```python
from build123d import *

# Parameters (mm, degrees)
F1_DEPTH = 25.4
F2_R     = 2.486175
F3_DEPTH = 25.4


with BuildPart() as f1:
    # F0 (on Top) → F1 (new body)
    with BuildSketch(Plane.XY):
        Polygon((-25.4, 0), (0, 0), (-25.4, 33.05722), align=None)
    extrude(amount=F1_DEPTH)

    # F2 (on face) → F3 (join)
    with BuildSketch(Plane.XY.offset(25.4)):
        with Locations((-16.399799, 11.118355)):
            Circle(F2_R)
    extrude(amount=F3_DEPTH)


solid = f1.part
```
Work out the finished part from the listing and answer in its coordinate system (mm). Give positions to 0.01 mm unless a question says otherwise; leave off trailing zeros. Loops run counter-clockwise (first coordinate to the right, second up) from the corner with the lowest first, then second, coordinate; pieces in that order, holes last. Notation, with made-up numbers: (-6.5, 63) - (14.5, 63) arc R13 cw to (14.5, 75) - close; hole circle Ø6 at (88, -22.5). An arc over 180 degrees is marked (long way). Use CSV: the item, a comma, the result in double quotes. Start each with the question number.
(1) Find section A-A, the plane y = 10. Determine the outline of the cut face in (x, z), plus the area to 3 significant figures.
(2) Find section D-D, the plane y = 21. Determine the outline of the cut face in (x, z), plus the area to 3 significant figures.
(3) This flat-tipped pin is pushed along its axis until it touches: pin 1 (6 mm diameter, centred on x = -15, y = 22, fed in from +Z). Where does it stop, or does it pass through?
(4) Find section B-B, the plane x = -17. Determine the outline of the cut face in (y, z).
(5) Determine the mould class of faces 1 (the face through (-13, 0, 13)), 2 (the face through (-12.522, 16.297, 12.522)), 3 (the face through (-14.1, 10.17, 37.92)) for opening direction X: released by +X, released by -X, zero draft, split by the parting line, or undercut.
(6) Find section C-C, the plane z = 21. Determine the outline of the cut face in (x, y), plus the area to 3 significant figures.
(7) Find the intervals of material crossed by L1, parallel to Z at x = -9.5, y = 5.5; L2, parallel to X at y = 10, z = 40.5; L3, parallel to Y at x = -20.75, z = 15.5, in increasing order.
Results found:
1,outline,"(-25.4, 0) - (-7.68, 0) - (-7.68, 25.4) - (-14.18, 25.4) - (-14.18, 50.8) - (-18.62, 50.8) - (-18.62, 25.4) - (-25.4, 25.4) - close"
1,area,"563 mm^2"
2,outline,"(-25.4, 0) - (-16.14, 0) - (-16.14, 25.4) - (-25.4, 25.4) - close"
2,area,"235 mm^2"
3,pin 1,"z = 25.4"
4,outline,"(0, 0) - (22.12, 0) - (22.12, 25.4) - (13.53, 25.4) - (13.53, 50.8) - (8.71, 50.8) - (8.71, 25.4) - (0, 25.4) - close"
5,face 1,"zero draft"
5,face 2,"released by +X"
5,face 3,"split by the parting line"
6,outline,"(-25.4, 0) - (0, 0) - (-25.4, 33.06) - close"
6,area,"420 mm^2"
7,L1,"0 to 25.4"
7,L2,"-18.62 to -14.18"
7,L3,"0 to 27.01"
